```python
from build123d import *

# Parameters (mm, degrees)
SKETCH1_W           = 25.41
SKETCH1_H           = 12
BOSS_EXTRUDE1_DEPTH = 6
SKETCH2_R           = 2.42
CUT_EXTRUDE1_DEPTH  = 25.41
SKETCH3_W           = 4.543452961
SKETCH3_H           = 1.5
CUT_EXTRUDE2_DEPTH  = 25.41
SKETCH4_R           = 0.8
CUT_EXTRUDE4_DEPTH  = 7


with BuildPart() as part:
    # Sketch1 → Boss-Extrude1 (new body)
    with BuildSketch(Plane(origin=(0, 0, 0), x_dir=(1, 0, 0), z_dir=(0, 1, 0))):
        with Locations((12.705, 6)):
            Rectangle(SKETCH1_W, SKETCH1_H)
    extrude(amount=BOSS_EXTRUDE1_DEPTH)

    # Sketch2 → Cut-Extrude1 (cut)
    with BuildSketch(Plane.ZY):
        with Locations((-6, 6)):
            Circle(SKETCH2_R)
    extrude(amount=-CUT_EXTRUDE1_DEPTH, mode=Mode.SUBTRACT)

    # Sketch3 → Cut-Extrude2 (cut)
    with BuildSketch(Plane.ZY):
        with Locations((-9.72827352, 5.25)):
            Rectangle(SKETCH3_W, SKETCH3_H)
    extrude(amount=-CUT_EXTRUDE2_DEPTH, mode=Mode.SUBTRACT)

    # Sketch4 → Cut-Extrude4 (cut, through all)
    with BuildSketch(Plane(origin=(0, 6, 0), x_dir=(1, 0, 0), z_dir=(0, 1, 0))):
        with Locations((5.082, 1.79)):
            Circle(SKETCH4_R)
        with Locations((10.164, 1.79)):
            Circle(SKETCH4_R)
        with Locations((15.246, 1.79)):
            Circle(SKETCH4_R)
        with Locations((20.328, 1.79)):
            Circle(SKETCH4_R)
    extrude(amount=-CUT_EXTRUDE4_DEPTH, mode=Mode.SUBTRACT)


solid = part.part
```
Geometry: final body of the model. Coordinates: model frame, mm. A direction names the side the tool comes from. Round coordinates to 2 decimals unless told otherwise and drop trailing zeros. Loops run counter-clockwise (first coordinate to the right, second up) from the corner with the lowest first, then second, coordinate; pieces in that order, holes last.
Item 1: Section A-A, the plane y = 1.9. Output: boundary loops of the cut face in (x, z), plus the area to 3 significant figures.
Checked values:
outline: (0, -12) - (25.41, -12) - (25.41, 0) - (0, 0) - close; hole circle Ø1.6 at (5.08, -1.79); hole circle Ø1.6 at (10.16, -1.79); hole circle Ø1.6 at (15.25, -1.79); hole circle Ø1.6 at (20.33, -1.79)
area: 297 mm2
Item 2: Reachability of faces 1 (the cylindrical face through (16.01, 3.04, -2.03)), 2 (the flat face through (13, 4.5, -10)) from +Z, -Z, +X, -X, +Y, -Y: full face, straight path, thin tool, end or side. Return the list, or none.
Checked values:
face 1: +Y, -Y
face 2: -Z, +X, -X, +Y
Item 3: Contact query for flat-ended pins moving along their axis: P1, Ø3.5, axis at x = 17, z = -11, coming from the +Y side; P2, Ø1.8, axis at x = 20.328, z = -1.79, coming from the -Y side. Output: stop coordinate, or through.
Checked values:
P1: stops at y = 4.5
P2: stops at y = 0
Item 4: Line query: L1, parallel to X at y = 1.8, z = -1.79; L2, parallel to X at y = 2.55, z = -2.25; L3, parallel to Z at x = 20.25, y = 2.25. Output: solid intervals per line, ascending.
Checked values:
L1: x = 0 to 4.28, 5.88 to 9.36, 10.96 to 14.45, 16.05 to 19.53, 21.13 to 25.41
L2: x = 0 to 4.43, 5.74 to 9.51, 10.82 to 14.59, 15.9 to 19.67, 20.98 to 25.41
L3: z = -12 to -2.59, -0.99 to 0
Item 5: Section D-D, the plane x = 7. Output: boundary loops of the cut face in (y, z), plus the area to 3 significant figures.
Checked values:
outline: (0, -12) - (4.5, -12) - (4.5, -7.9) arc R2.42 cw to (6, -3.58) - (6, 0) - (0, 0) - close
area: 57.2 mm2
Item 6: Section B-B, the plane z = -1.25. Output: boundary loops of the cut face in (x, y), plus the area to 3 significant figures.
Checked values:
outline: (0, 0) - (4.49, 0) - (4.49, 6) - (0, 6) - close; (5.67, 0) - (9.57, 0) - (9.57, 6) - (5.67, 6) - close; (10.75, 0) - (14.66, 0) - (14.66, 6) - (10.75, 6) - close; (15.84, 0) - (19.74, 0) - (19.74, 6) - (15.84, 6) - close; (20.92, 0) - (25.41, 0) - (25.41, 6) - (20.92, 6) - close
area: 124 mm2
Item 7: Mould query, pull axis Z, two halves, no side actions, for faces 3 (the flat face through (13, 2, -12)), 4 (the cylindrical face through (21.1, 3, -2)), 5 (the flat face through (13, 3, 0)). Classes: released by +Z, released by -Z, zero draft, split by the parting line, or undercut.
Checked values:
face 3: released by -Z
face 4: undercut
face 5: released by +Z
Item 8: Section C-C, the plane x = 15.25. Output: boundary loops of the cut face in (y, z), plus the area to 3 significant figures.
Checked values:
outline: (0, -12) - (4.5, -12) - (4.5, -7.9) arc R2.42 cw to (6, -3.58) - (6, -2.59) - (0, -2.59) - close; (0, -0.99) - (6, -0.99) - (6, 0) - (0, 0) - close
area: 47.6 mm2
